Here's how the part is built. I have some questions about the finished solid (model axes, mm). Face numbers are marked on the shaded views. A direction names the side the tool comes from. Round coordinates to 2 decimals unless told otherwise and drop trailing zeros. Order: outer loops, then holes, each group sorted by start corner. A loop starts at its lowest first (then second) coordinate and runs counter-clockwise, first axis right, second up. Notation, with made-up numbers: (24, 72) - (79, 72) arc R20 cw to (79, 85) - close; hole circle Ø3 at (33.5, 18.25). An arc over 180 degrees is marked (long way). Answer as a JSON object with one key per item and string values.
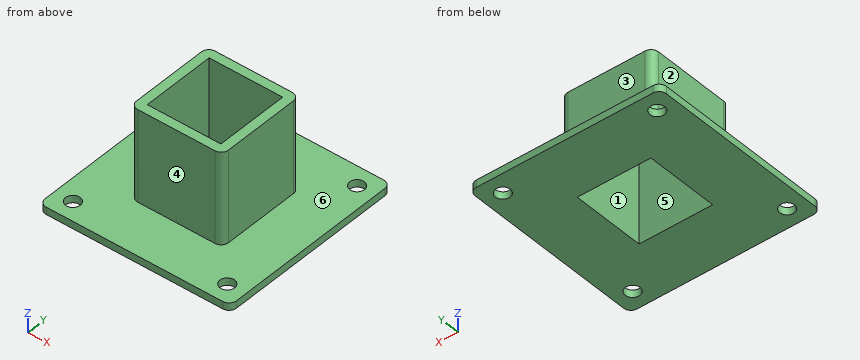
```python
from build123d import *

# Parameters (mm, degrees)
SKETCH_1_W          = 25
SKETCH_1_H          = 25
SKETCH_1_W_2        = 20
SKETCH_1_H_2        = 20
EXTRUDE_1_DEPTH     = 25
SKETCH_3_W          = 52
SKETCH_3_H          = 52
EXTRUDE_2_DEPTH     = 2
SKETCH_4_W          = 20
SKETCH_4_H          = 20
CUT_EXTRUDE_1_DEPTH = 28
FILLET_1_R          = 2
FILLET_2_R          = 2
FILLET_3_R          = 2
FILLET_4_R          = 2
FILLET_5_R          = 2
FILLET_6_R          = 2
FILLET_7_R          = 2
FILLET_8_R          = 2
SKETCH_5_R          = 2
CUT_EXTRUDE_2_DEPTH = 28


with BuildPart() as part:
    # 草图1 → 凸台-拉伸1 (new body)
    with BuildSketch(Plane.XY):
        Rectangle(SKETCH_1_W, SKETCH_1_H)
        Rectangle(SKETCH_1_W_2, SKETCH_1_H_2, mode=Mode.SUBTRACT)
    extrude(amount=EXTRUDE_1_DEPTH)

    # 草图3 → 凸台-拉伸2 (add)
    with BuildSketch(Plane(origin=(0, 0, 0), x_dir=(-1, 0, 0), z_dir=(0, 0, -1))):
        Rectangle(SKETCH_3_W, SKETCH_3_H)
    extrude(amount=EXTRUDE_2_DEPTH)

    # 草图4 → 切除-拉伸1 (cut, through all)
    with BuildSketch(Plane(origin=(0, 0, -2), x_dir=(-1, 0, 0), z_dir=(0, 0, -1))):
        Rectangle(SKETCH_4_W, SKETCH_4_H)
    extrude(amount=-CUT_EXTRUDE_1_DEPTH, mode=Mode.SUBTRACT)

    # 圆角1
    fillet_1_edges = [part.edges().sort_by_distance(p)[0] for p in [
        (-26, 26, -1),
    ]]
    fillet(fillet_1_edges, radius=FILLET_1_R)

    # 圆角2
    fillet_2_edges = [part.edges().sort_by_distance(p)[0] for p in [
        (-26, -26, -1),
    ]]
    fillet(fillet_2_edges, radius=FILLET_2_R)

    # 圆角3
    fillet_3_edges = [part.edges().sort_by_distance(p)[0] for p in [
        (26, -26, -1),
    ]]
    fillet(fillet_3_edges, radius=FILLET_3_R)

    # 圆角4
    fillet_4_edges = [part.edges().sort_by_distance(p)[0] for p in [
        (26, 26, -1),
    ]]
    fillet(fillet_4_edges, radius=FILLET_4_R)

    # 圆角5
    fillet_5_edges = [part.edges().sort_by_distance(p)[0] for p in [
        (-12.5, -12.5, 12.5),
    ]]
    fillet(fillet_5_edges, radius=FILLET_5_R)

    # 圆角6
    fillet_6_edges = [part.edges().sort_by_distance(p)[0] for p in [
        (-12.5, 12.5, 12.5),
    ]]
    fillet(fillet_6_edges, radius=FILLET_6_R)

    # 圆角7
    fillet_7_edges = [part.edges().sort_by_distance(p)[0] for p in [
        (12.5, 12.5, 12.5),
    ]]
    fillet(fillet_7_edges, radius=FILLET_7_R)

    # 圆角8
    fillet_8_edges = [part.edges().sort_by_distance(p)[0] for p in [
        (12.5, -12.5, 12.5),
    ]]
    fillet(fillet_8_edges, radius=FILLET_8_R)

    # 草图5 → 切除-拉伸2 (cut, through all)
    with BuildSketch(Plane(origin=(0, 0, -2), x_dir=(-1, 0, 0), z_dir=(0, 0, -1))):
        with Locations((-21, 21)):
            Circle(SKETCH_5_R)
        with Locations((21, 21)):
            Circle(SKETCH_5_R)
        with Locations((-21, -21)):
            Circle(SKETCH_5_R)
        with Locations((21, -21)):
            Circle(SKETCH_5_R)
    extrude(amount=-CUT_EXTRUDE_2_DEPTH, mode=Mode.SUBTRACT)


solid = part.part
```
1. Imagine slicing it at C-C (y = 21). List the corners of the cut face in (x, z) for me, plus the area to 3 significant figures.
Responses:
{"outline": "(-26, -2) - (-23, -2) - (-23, 0) - (-26, 0) - close; (-19, -2) - (19, -2) - (19, 0) - (-19, 0) - close; (23, -2) - (26, -2) - (26, 0) - (23, 0) - close", "area": "88.0 mm2"}
2. Imagine slicing it at B-B (z = 13.25). List the corners of the cut face in (x, y) for me, plus the area to 3 significant figures.
Responses:
{"outline": "(-12.5, -10.5) arc R2 ccw to (-10.5, -12.5) - (10.5, -12.5) arc R2 ccw to (12.5, -10.5) - (12.5, 10.5) arc R2 ccw to (10.5, 12.5) - (-10.5, 12.5) arc R2 ccw to (-12.5, 10.5) - close; hole (-10, -10) - (10, -10) - (10, 10) - (-10, 10) - close", "area": "222 mm2"}
3. If I drill on L1, parallel to Y at x = 21, z = -0.65; L2, parallel to X at y = 4, z = 19.75; L3, parallel to Z at x = -22, y = -16.5, over which ranges is the centre line in solid material (lowest first)? Write a range as [from, to].
Responses:
{"L1": "[-26, -23], [-19, 19], [23, 26]", "L2": "[-12.5, -10], [10, 12.5]", "L3": "[-2, 0]"}
4. Thinking about a two-plate mould opening in Y: for the marked faces 1, 2 and 3, which applies, pulls with the +Y half, pulls with the -Y half, needs draft (parallel to the pull), parting line crosses it, or undercut?
Responses:
{"face 1": "undercut", "face 2": "needs draft", "face 3": "pulls with the +Y half"}
5. For P1, Ø16, axis at y = 3, z = 15.5, coming from the -X side; P2, Ø4.5, axis at x = -21, y = 21, coming from the -Z side; P3, Ø12, axis at x = 4, z = 14.5, coming from the -Y side; P4, Ø1.5, axis at x = -17, y = 18, coming from the +Z side, each with a flat end and sliding along its axis, tell me the tip position at first contact or that it passes through.
Responses:
{"P1": "x = -12.5", "P2": "z = -2", "P3": "y = -12.5", "P4": "z = 0"}
6. For the marked faces 4, 5 and 6, which set-ups out of +Z, -Z, +X, -X, +Y, -Y let a thin tool reach every point of the face, with its end or its side?
Responses:
{"face 4": "+Z, +X, -X, -Y", "face 5": "+Z, -Z", "face 6": "+Z"}
7. Imagine slicing it at A-A (x = 5). List the corners of the cut face in (y, z) for me.
Responses:
{"outline": "(-26, -2) - (-10, -2) - (-10, 25) - (-12.5, 25) - (-12.5, 0) - (-26, 0) - close; (10, -2) - (26, -2) - (26, 0) - (12.5, 0) - (12.5, 25) - (10, 25) - close"}
